from build123d import *

# Parameters (mm, degrees)
SKETCH1_R           = 32.5
SKETCH1_R_2         = 11.5
SKETCH1_R_3         = 2.6
BOSS_EXTRUDE1_DEPTH = 16
SKETCH2_R           = 20
CUT_EXTRUDE1_DEPTH  = 11


with BuildPart() as part:
    # Sketch1 → Boss-Extrude1 (new body)
    with BuildSketch(Plane(origin=(0, 0, 0), x_dir=(1, 0, 0), z_dir=(0, 1, 0))):
        with Locations(Location((0, 0, 0), (0, 0, 270))):
            Circle(SKETCH1_R)
        with Locations(Location((0, 0, 0), (0, 0, 270))):
            Circle(SKETCH1_R_2, mode=Mode.SUBTRACT)
        with Locations(Location((18.384776311, -18.384776311, 0), (0, 0, 270))):
            Circle(SKETCH1_R_3, mode=Mode.SUBTRACT)
        with Locations(Location((-18.384776311, -18.384776311, 0), (0, 0, 270))):
            Circle(SKETCH1_R_3, mode=Mode.SUBTRACT)
        with Locations(Location((-18.384776311, 18.384776311, 0), (0, 0, 270))):
            Circle(SKETCH1_R_3, mode=Mode.SUBTRACT)
        with Locations(Location((18.384776311, 18.384776311, 0), (0, 0, 270))):
            Circle(SKETCH1_R_3, mode=Mode.SUBTRACT)
    extrude(amount=BOSS_EXTRUDE1_DEPTH)

    # Sketch2 → Cut-Extrude1 (cut)
    with BuildSketch(Plane(origin=(0, 16, 0), x_dir=(1, 0, 0), z_dir=(0, 1, 0))):
        with Locations(Location((0, 0, 0), (0, 0, 270))):
            Circle(SKETCH2_R)
    extrude(amount=-CUT_EXTRUDE1_DEPTH, mode=Mode.SUBTRACT)


solid = part.part
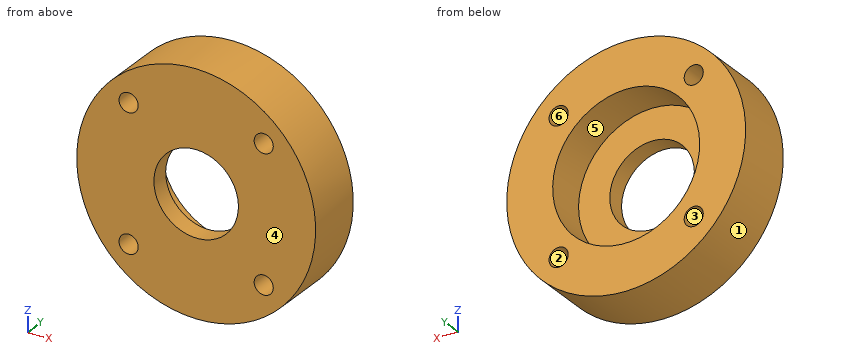
The listing builds one solid part. Answer for the finished solid, in the listing's coordinates (mm). Face numbers are marked on the shaded views. A direction names the side the tool comes from. Coordinates: 2 decimals unless noted, no trailing zeros. Write each loop counter-clockwise with the first axis right and the second up, starting at its lowest first coordinate (ties: lowest second). Pieces come first, ordered by that corner, then holes. Notation, with made-up numbers: (-34, 58) -> (6, 58) arc R29 cw to (6, 87) -> close; hole circle Ø11 at (7, -21.75). An arc over 180 degrees is marked (long way). One line per question, with ' | ' between items.
1. Section A-A (x = 0) is taken. Determine the outline of the cut face in (y, z), and give its area (3 significant figures).
Verdict:
outline: (0, -32.5) -> (16, -32.5) -> (16, -20) -> (5, -20) -> (5, -11.5) -> (0, -11.5) -> close; (0, 11.5) -> (5, 11.5) -> (5, 20) -> (16, 20) -> (16, 32.5) -> (0, 32.5) -> close | area: 485 mm^2
2. Straight lines are drawn through the part: line 1 (Z direction, x = 16, y = 2); line 2 (Z direction, x = 18, y = 10.75); line 3 (X direction, y = 15.75, z = 20.5). For each, find the intervals that lie inside material, in ascending order.
Verdict:
line 1: z = -28.29 to -19.42, -17.35 to 17.35, 19.42 to 28.29 | line 2: z = -27.06 to -20.96, -15.81 to -8.72, 8.72 to 15.81, 20.96 to 27.06 | line 3: x = -25.22 to -19.9, -16.87 to 16.87, 19.9 to 25.22
3. For a pull along X with two mould halves and no side action, classify the marked faces 1, 2, 3 and 4 as released by +X, released by -X, zero draft, split by the parting line, or undercut.
Verdict:
face 1: split by the parting line | face 2: undercut | face 3: undercut | face 4: zero draft
4. Section D-D (z = 17) is taken. Determine the outline of the cut face in (x, y), and give its area (3 significant figures).
Verdict:
outline: (-27.7, 0) -> (-20.59, 0) -> (-20.59, 16) -> (-27.7, 16) -> close; (-16.18, 0) -> (16.18, 0) -> (16.18, 16) -> (10.54, 16) -> (10.54, 5) -> (-10.54, 5) -> (-10.54, 16) -> (-16.18, 16) -> close; (20.59, 0) -> (27.7, 0) -> (27.7, 16) -> (20.59, 16) -> close | area: 514 mm^2
5. Section C-C (y = 13) is taken. Determine the outline of the cut face in (x, z).
Verdict:
outline: circle Ø65 at (0, 0); hole circle Ø5.2 at (-18.38, -18.38); hole circle Ø5.2 at (-18.38, 18.38); hole circle Ø40 at (0, 0); hole circle Ø5.2 at (18.38, -18.38); hole circle Ø5.2 at (18.38, 18.38)
6. Which of the six approach directions +Z, -Z, +X, -X, +Y, -Y give full straight-line access (tool end or side, diameter ignored) to the marked faces 5 and 6?
Verdict:
face 5: +Y | face 6: +Y, -Y
7. Section B-B (z = 0) is taken. Determine the outline of the cut face in (x, y), and give its area (3 significant figures).
Verdict:
outline: (-32.5, 0) -> (-11.5, 0) -> (-11.5, 5) -> (-20, 5) -> (-20, 16) -> (-32.5, 16) -> close; (11.5, 0) -> (32.5, 0) -> (32.5, 16) -> (20, 16) -> (20, 5) -> (11.5, 5) -> close | area: 485 mm^2
8. Given pin 1 Ø4 at (y, z) = (1.5, -21) entering from +X; pin 2 Ø8.5 at (x, z) = (18.38, 18.38) entering from -Y; pin 3 Ø1 at (y, z) = (12, -21.5) entering from +X; pin 4 Ø1.5 at (x, z) = (-10.5, 7.5) entering from +Y, each flat-ended and moving along its own axis, determine where each tip first touches the part or whether it passes through.
Verdict:
pin 1: stops at x = 26.37 | pin 2: stops at y = 0 | pin 3: stops at x = 24.8 | pin 4: stops at y = 5
